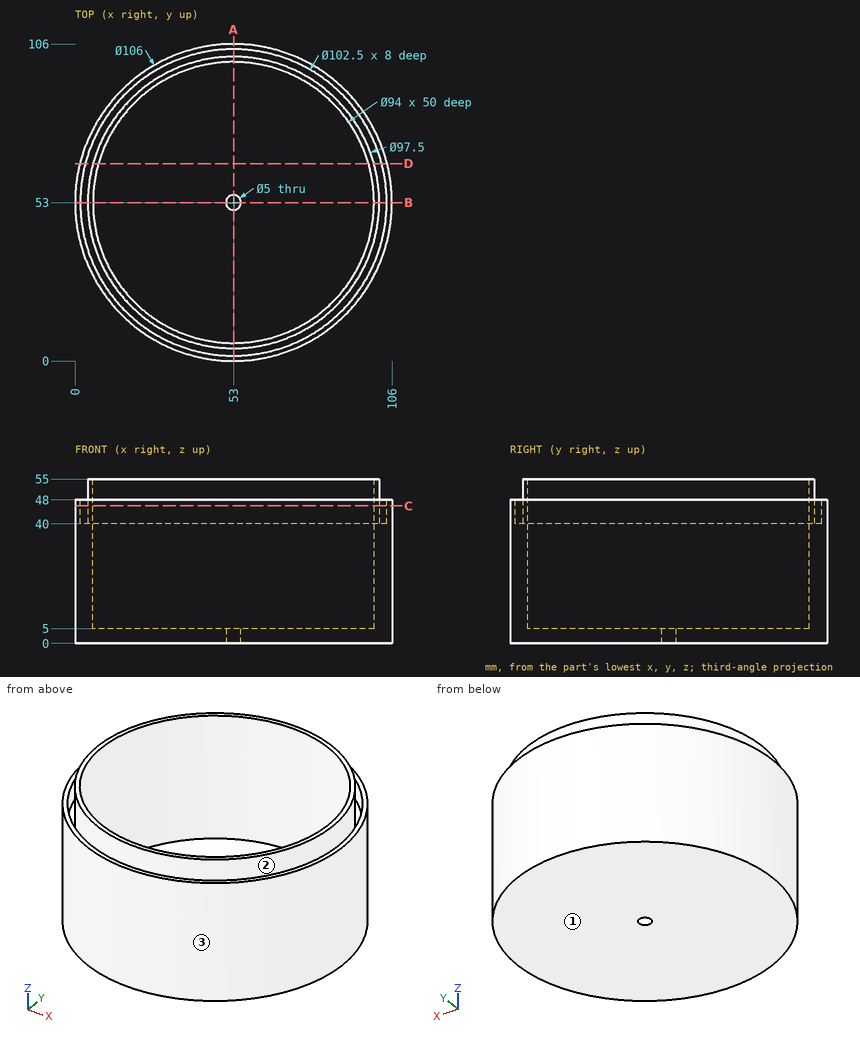
Input: dimensioned drawing with shaded views. Units: mm. Origin: part minimum x, y, z. Give positions to 0.01 mm unless a question says otherwise; leave off trailing zeros. Write each loop counter-clockwise with the first axis right and the second up, starting at its lowest first coordinate (ties: lowest second). Pieces come first, ordered by that corner, then holes.
1. Material intervals for line 1 along Y through (x, z) = (53, 44.75); line 2 along Y through (x, z) = (53, 2.45); line 3 along Y through (x, z) = (67, 41), sorted ascending.
2. Section query D-D (y = 66). Return the cut outline in (x, z).
3. Section query C-C (z = 46). Return the cut outline in (x, y), then the cut area to 3 significant figures.
4. First-contact query: pin 1 (2 mm diameter, centred on y = 12.5, z = 33, fed in from +X); pin 2 (1.5 mm diameter, centred on x = 57.5, z = 16, fed in from -Y); pin 3 (4.5 mm diameter, centred on x = 53, y = 53, fed in from -Z); pin 4 (2 mm diameter, centred on x = 43, z = 22, fed in from +Y). Flat tips, straight axial feed; report the tip coordinate or a pass-through.
5. Section query A-A (x = 53). Return the cut outline in (y, z), then the cut area to 3 significant figures.
6. Pull-direction query (X, two-part tool) for the marked faces 1, 2 and 3; classes: +X half, -X half, draft (parallel to the pull), parting line (faces both ways), or undercut.
Output values:
1. line 1: y = 0 to 1.75, 4.25 to 6, 100 to 101.75, 104.25 to 106
1. line 2: y = 0 to 50.5, 55.5 to 106
1. line 3: y = 1.88 to 3.7, 6.3 to 8.13, 97.87 to 99.7, 102.3 to 104.12
2. outline: (1.62, 0) - (104.38, 0) - (104.38, 48) - (102.57, 48) - (102.57, 40) - (99.98, 40) - (99.98, 55) - (98.17, 55) - (98.17, 5) - (7.83, 5) - (7.83, 55) - (6.02, 55) - (6.02, 40) - (3.43, 40) - (3.43, 48) - (1.62, 48) - close
3. outline: circle Ø106 at (53, 53); circle Ø97.5 at (53, 53); hole circle Ø102.5 at (53, 53); hole circle Ø94 at (53, 53)
3. area: 1,100 mm2
4. pin 1: stops at x = 88.34
4. pin 2: stops at y = 0.13
4. pin 3: passes through
4. pin 4: stops at y = 105.23
5. outline: (0, 0) - (50.5, 0) - (50.5, 5) - (6, 5) - (6, 55) - (4.25, 55) - (4.25, 40) - (1.75, 40) - (1.75, 48) - (0, 48) - close; (55.5, 0) - (106, 0) - (106, 48) - (104.25, 48) - (104.25, 40) - (101.75, 40) - (101.75, 55) - (100, 55) - (100, 5) - (55.5, 5) - close
5. area: 1,010 mm2
6. face 1: draft
6. face 2: undercut
6. face 3: parting line
